```python
from build123d import *

# Parameters (mm, degrees)
BOX_W               = 313
BOX_H               = 200
BOX_DEPTH           = 37
BOX_PLACEMENT_ANGLE = 45
BOX008_W            = 200
BOX008_H            = 200
BOX008_DEPTH        = 33


with BuildPart() as cube002:
    # Box → Box (new body)
    with BuildSketch(Plane.XY):
        with Locations((156.5, 100)):
            Rectangle(BOX_W, BOX_H)
    extrude(amount=BOX_DEPTH)


with BuildPart() as cube002_1:
    # Box placement: moved
    add(cube002.part.moved(Location((0, 0, -2))).rotate(Axis((0, 0, -2), (0, 0, 1)), BOX_PLACEMENT_ANGLE))


with BuildPart() as long_45a:
    # Box008 → Box008 (new body)
    with BuildSketch(Plane.XY.offset(-1)):
        with Locations((100, 100)):
            Rectangle(BOX008_W, BOX008_H)
    extrude(amount=BOX008_DEPTH)

    # Cut006: cut Cube002
    add(cube002_1.part, mode=Mode.SUBTRACT)


solid = long_45a.part
```
Check sheet for the modelled part. Datum: model origin and axes. Units: mm. Round coordinates to 2 decimals unless told otherwise and drop trailing zeros. Order: outer loops, then holes, each group sorted by start corner. A loop starts at its lowest first (then second) coordinate and runs counter-clockwise, first axis right, second up.
1) Section check B-B (x = 50). Record the boundary of the cut face in (y, z).
2) Section check A-A (y = 47.5). Record the boundary of the cut face in (x, z).
3) Go/stop test with flat-tipped pins: pin 1 Ø6 at (x, z) = (123.5, 26) entering from +Y; pin 2 Ø10 at (y, z) = (41.5, 10.5) entering from -X; pin 3 Ø5 at (y, z) = (84, 26.5) entering from -X. Record where each tip stops, or that it passes through.
4) Scan lines: line 1 (Y direction, x = 165, z = 9); line 2 (X direction, y = 46, z = 27); line 3 (X direction, y = 109.5, z = 10). Record each from-to range of solid material in increasing order.
5) Section check C-C (z = 11.5). Record the boundary of the cut face in (x, y), and give its area (3 significant figures).
Result:
1. outline: (0, -1) - (50, -1) - (50, 32) - (0, 32) - close
2. outline: (47.5, -1) - (200, -1) - (200, 32) - (47.5, 32) - close
3. pin 1: stops at y = 126.5
3. pin 2: stops at x = 36.5
3. pin 3: stops at x = 81.5
4. line 1: y = 0 to 165
4. line 2: x = 46 to 200
4. line 3: x = 109.5 to 200
5. outline: (0, 0) - (200, 0) - (200, 200) - close
5. area: 20,000 mm2
